Can you work these out from the model? Positions are in its coordinate system, mm. A direction names the side the tool comes from. Give positions to 0.01 mm unless a question says otherwise; leave off trailing zeros. Write each loop counter-clockwise with the first axis right and the second up, starting at its lowest first coordinate (ties: lowest second). Pieces come first, ordered by that corner, then holes.
from build123d import *

# Parameters (mm, degrees)
SKETCH2_W                      = 19
SKETCH2_H                      = 20
BOSS_EXTRUDE1_DEPTH            = 7.5
F_3_7_3_7_DIAMETER_HOLE2_D     = 3.7
F_3_7_3_7_DIAMETER_HOLE2_DEPTH = 11.6
F_3_7_3_7_DIAMETER_HOLE2_TIP   = 1.111592145
SKETCH10_W                     = 20
SKETCH10_H                     = 8
BOSS_EXTRUDE2_DEPTH            = 3
F_3_7_3_7_DIAMETER_HOLE1_D     = 3.7


with BuildPart() as part:
    # Sketch2 → Boss-Extrude1 (new, symmetric)
    with BuildSketch(Plane(origin=(0, 0, 0), x_dir=(1, 0, 0), z_dir=(0, 1, 0))):
        Rectangle(SKETCH2_W, SKETCH2_H)
    extrude(amount=BOSS_EXTRUDE1_DEPTH, both=True)

    # Ø3.7 (3.7) Diameter Hole2
    with Locations(Plane.ZY.offset(9.5)):
        with Locations((-5, -3.5), (5, -3.5)):
            Hole(F_3_7_3_7_DIAMETER_HOLE2_D / 2, depth=F_3_7_3_7_DIAMETER_HOLE2_DEPTH)
            with Locations((0, 0, -(F_3_7_3_7_DIAMETER_HOLE2_DEPTH + F_3_7_3_7_DIAMETER_HOLE2_TIP / 2))):  # 118° drill point
                Cone(0, F_3_7_3_7_DIAMETER_HOLE2_D / 2, F_3_7_3_7_DIAMETER_HOLE2_TIP, mode=Mode.SUBTRACT)

    # Sketch10 → Boss-Extrude2 (add)
    with BuildSketch(Plane.ZY.offset(9.5)):
        with Locations((0, 3.5)):
            Rectangle(SKETCH10_W, SKETCH10_H)
    extrude(amount=BOSS_EXTRUDE2_DEPTH)

    # Ø3.7 (3.7) Diameter Hole1 (through all)
    with Locations(Plane(origin=(0, 0, -10), x_dir=(-1, 0, 0), z_dir=(0, 0, -1))):
        with Locations((6.25, 2.5)):
            Hole(F_3_7_3_7_DIAMETER_HOLE1_D / 2)


solid = part.part
(1) Imagine slicing it at B-B, the plane z = 0. Write out the boundary of the cut face in (x, y).
Returned:
outline: (-12.5, -0.5) - (-9.5, -0.5) - (-9.5, -7.5) - (9.5, -7.5) - (9.5, 7.5) - (-12.5, 7.5) - close; hole circle Ø3.7 at (-6.25, 2.5)
(2) Imagine slicing it at A-A, the plane x = -6.25. Write out the boundary of the cut face in (y, z), plus the area to 3 significant figures.
Returned:
outline: (-7.5, -10) - (0.65, -10) - (0.65, 10) - (-7.5, 10) - close; (4.35, -10) - (7.5, -10) - (7.5, 10) - (4.35, 10) - close; hole circle Ø3.7 at (-3.5, -5); hole circle Ø3.7 at (-3.5, 5)
area: 204 mm2
(3) Will these pins go through, and if not, where does the flat tip stop? P1, Ø2, axis at y = -3.5, z = 5, coming from the -X side; P2, Ø2, axis at x = -6.25, y = 2.5, coming from the -Z side.
Returned:
P1: stops at x = 2.61
P2: passes through
(4) If I drill on L1, parallel to Y at x = -6.25, z = 5; L2, parallel to Y at x = -2.25, z = 5; L3, parallel to Z at x = -3, y = -3.5, over which ranges is the centre line in solid material (lowest first)?
Returned:
L1: y = -7.5 to -5.35, -1.65 to 0.65, 4.35 to 7.5
L2: y = -7.5 to -5.35, -1.65 to 7.5
L3: z = -10 to -6.85, -3.15 to 3.15, 6.85 to 10
(5) If we mould it in two halves opening along Y, with no side actions, what happens to faces 1 (the face through (-3.62, -3.42, 6.85)), 2 (the face through (-8.1, 2.58, 0.14)), 3 (the face through (-11, -0.5, 0)), 4 (the face through (-9.5, -4, 0))? For each: +Y half, -Y half, draft (parallel to the pull), parting line (faces both ways), or undercut.
Returned:
face 1: undercut
face 2: undercut
face 3: -Y half
face 4: draft
(6) For faces 5 (the face through (-3.62, -3.42, -3.15)), 6 (the face through (-1, 0, 10)), which set-ups out of +Z, -Z, +X, -X, +Y, -Y let a thin tool reach every point of the face, with its end or its side?
Returned:
face 5: -X
face 6: +Z, +X, -X, +Y, -Y
(7) Imagine slicing it at C-C, the plane y = 2. Write out the boundary of the cut face in (x, z), plus the area to 3 significant figures.
Returned:
outline: (-12.5, -10) - (-8.03, -10) - (-8.03, 10) - (-12.5, 10) - close; (-4.47, -10) - (9.5, -10) - (9.5, 10) - (-4.47, 10) - close
area: 369 mm2
(8) Imagine slicing it at D-D, the plane y = -1.25. Write out the boundary of the cut face in (x, z), plus the area to 3 significant figures.
Returned:
outline: (-9.5, -10) - (9.5, -10) - (9.5, 10) - (-9.5, 10) - close
area: 380 mm2
